from build123d import *

# Parameters (mm, degrees)
RING_SKETCH_W          = 18
RING_SKETCH_H          = 10
BUSHING_BORE_SKETCH_W  = 4
BUSHING_BORE_SKETCH_H  = 12
BUSHING_BORES_X4_COUNT = 4


with BuildPart() as part:
    # Ring Sketch → Ring (revolve)
    with BuildSketch(Plane.XY, mode=Mode.PRIVATE) as ring_sk:
        with Locations((-48, 85)):
            Rectangle(RING_SKETCH_W, RING_SKETCH_H)
    revolve(ring_sk.sketch.rotate(Axis((-108, 0, 0), (1, 0, 0)), 90), axis=Axis((-108, 0, 0), (1, 0, 0)))

    # Bushing Bore Sketch → Bushing Bore (revolve, cut)
    with BuildSketch(Plane.XY, mode=Mode.PRIVATE) as bushing_bore_sk:
        with Locations((-46, 85)):
            Rectangle(BUSHING_BORE_SKETCH_W, BUSHING_BORE_SKETCH_H)
    bushing_bore = revolve(bushing_bore_sk.sketch.rotate(Axis((-48, 70, 0), (0, 1, 0)), 90), axis=Axis((-48, 70, 0), (0, 1, 0)), mode=Mode.SUBTRACT)

    # Bushing Bores x4: Bushing Bore ×4 about axis
    bushing_bores_x4_axis = Axis((-38.1, 0, 0), (-1, 0, 0))
    for i in range(1, BUSHING_BORES_X4_COUNT):
        add(bushing_bore.rotate(bushing_bores_x4_axis, i * 360 / BUSHING_BORES_X4_COUNT), mode=Mode.SUBTRACT)


solid = part.part
Source: CAD feature listing. Evaluate the final solid. Frame: model axes, mm. Round coordinates to 2 decimals unless told otherwise and drop trailing zeros. Write each loop counter-clockwise with the first axis right and the second up, starting at its lowest first coordinate (ties: lowest second). Pieces come first, ordered by that corner, then holes. Notation, with made-up numbers: (46.5, -40) - (65.5, -40) arc R12 ccw to (65.5, -36) - close; hole circle Ø6 at (12.5, -19). An arc over 180 degrees is marked (long way). Use CSV: the item, a comma, the result in double quotes. Start each with the question number.
(1) Cut plane D-D, the plane y = 22. Return loops of the section in (x, z).
(2) Cut plane C-C, the plane z = 44. Return loops of the section in (x, y).
(3) Mould query, pull axis X, two halves, no side actions, for faces 1 (the face through (-44.451, 85.021, -1.846)), 2 (the face through (-57, 52.9, 60.4)), 3 (the face through (-39, 52.9, 60.4)). Classes: pulls with the +X half, pulls with the -X half, needs draft (parallel to the pull), parting line crosses it, or undercut.
(4) Cut plane A-A, the plane z = 0. Return loops of the section in (x, y).
(5) First-contact query: pin 1 Ø5 at (x, z) = (-50.5, -70) entering from +Y; pin 2 Ø10.5 at (x, y) = (-48, 0) entering from +Z; pin 3 Ø4 at (x, y) = (-45.5, -68) entering from +Z; pin 4 Ø3 at (x, y) = (-46.5, 14.5) entering from -Z. Flat tips, straight axial feed; report the tip coordinate or a pass-through.
(6) Material intervals for probe 1 along Y at (x, z) = (-42.5, -2) (3 decimals); probe 2 along X at (y, z) = (83.25, 0); probe 3 along Z at (x, y) = (-52, 43), sorted ascending. Write a range as [from, to].
Geometry says:
1,outline,"(-57, -87.27) - (-39, -87.27) - (-39, -76.92) - (-57, -76.92) - close; (-57, 76.92) - (-39, 76.92) - (-39, 87.27) - (-57, 87.27) - close"
2,outline,"(-57, -78.51) - (-39, -78.51) - (-39, -66.81) - (-57, -66.81) - close; (-57, 66.81) - (-39, 66.81) - (-39, 78.51) - (-57, 78.51) - close"
3,face 1,"undercut"
3,face 2,"pulls with the -X half"
3,face 3,"pulls with the +X half"
4,outline,"(-57, -90) - (-52, -90) - (-52, -80) - (-57, -80) - close; (-57, 80) - (-52, 80) - (-52, 90) - (-57, 90) - close; (-44, -90) - (-39, -90) - (-39, -80) - (-44, -80) - close; (-44, 80) - (-39, 80) - (-39, 90) - (-44, 90) - close"
5,pin 1,"y = 59.53"
5,pin 2,"z = 90"
5,pin 3,"z = 61.19"
5,pin 4,"z = -89.06"
6,probe 1,"[-89.978, -79.975], [79.975, 89.978]"
6,probe 2,"[-57, -52], [-44, -39]"
6,probe 3,"[-79.06, -67.46], [67.46, 79.06]"
